Design review of the part built by this model. Coordinates are the model's own, in mm. Face numbers are marked on the shaded views. A direction names the side the tool comes from. Coordinates: 2 decimals unless noted, no trailing zeros. Write each loop counter-clockwise with the first axis right and the second up, starting at its lowest first coordinate (ties: lowest second). Pieces come first, ordered by that corner, then holes. Notation, with made-up numbers: (44.5, 50) -> (71.5, 50) arc R28 cw to (71.5, 71) -> close; hole circle Ø3 at (2.25, 44). An arc over 180 degrees is marked (long way). Write item = value, one per line. Start each with the question number.
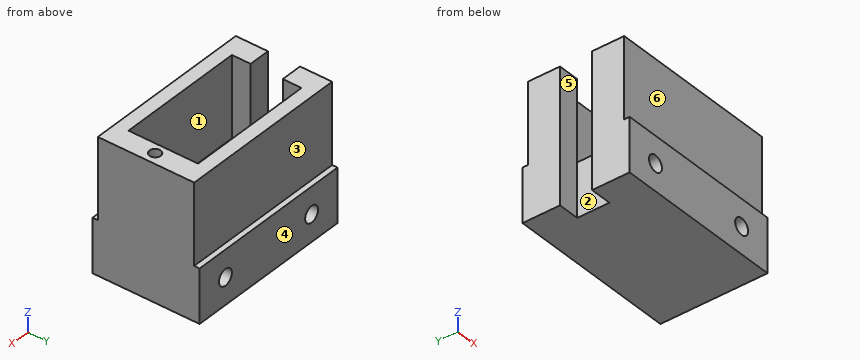
```python
from build123d import *

# Parameters (mm, degrees)
ESQUISSE15_W             = 32
ESQUISSE15_H             = 20
BOSS_EXTRU_1_DEPTH       = 10
ESQUISSE16_W             = 32
ESQUISSE16_H             = 18
ESQUISSE16_W_2           = 24
ESQUISSE16_H_2           = 13
BOSS_EXTRU_2_DEPTH       = 15
ESQUISSE17_W             = 25
ESQUISSE17_H             = 6
ENL_V_MAT_EXTRU_8_DEPTH  = 4
ESQUISSE19_R             = 1.05
ENL_V_MAT_EXTRU_10_DEPTH = 6
ENL_V_MAT_EXTRU_11_REACH = 22
ESQUISSE20_R             = 1.5


with BuildPart() as part:
    # Esquisse15 → Boss.-Extru.1 (new body)
    with BuildSketch(Plane.XY):
        Rectangle(ESQUISSE15_W, ESQUISSE15_H)
    extrude(amount=BOSS_EXTRU_1_DEPTH)

    # Esquisse16 → Boss.-Extru.2 (add)
    with BuildSketch(Plane.XY.offset(10)):
        Rectangle(ESQUISSE16_W, ESQUISSE16_H)
        Rectangle(ESQUISSE16_W_2, ESQUISSE16_H_2, mode=Mode.SUBTRACT)
    extrude(amount=BOSS_EXTRU_2_DEPTH)

    # Esquisse17 → Enlèv. mat.-Extru.8 (cut)
    with BuildSketch(Plane.ZY.offset(16)):
        with Locations((12.5, 0)):
            Rectangle(ESQUISSE17_W, ESQUISSE17_H)
    extrude(amount=-ENL_V_MAT_EXTRU_8_DEPTH, mode=Mode.SUBTRACT)

    # Esquisse19 → Enlèv. mat.-Extru.10 (cut)
    with BuildSketch(Plane.XY.offset(25)):
        with Locations((13.9, 0)):
            Circle(ESQUISSE19_R)
    extrude(amount=-ENL_V_MAT_EXTRU_10_DEPTH, mode=Mode.SUBTRACT)

    # Esquisse20 → Enlèv. mat.-Extru.11 (cut, up to next)
    with BuildSketch(Plane(origin=(0, 10, 0), x_dir=(1, 0, 0), z_dir=(0, 1, 0)), mode=Mode.PRIVATE) as enl_v_mat_extru_11_sk1:
        with Locations((-10, -5)):
            Circle(ESQUISSE20_R)
    enl_v_mat_extru_11_tool1 = extrude(enl_v_mat_extru_11_sk1.sketch, amount=-ENL_V_MAT_EXTRU_11_REACH, mode=Mode.PRIVATE) & part.part
    add(enl_v_mat_extru_11_tool1.solids().sort_by_distance((-10, 10, 5))[0], mode=Mode.SUBTRACT)
    # Esquisse20 → Enlèv. mat.-Extru.11 (cut, up to next)
    with BuildSketch(Plane(origin=(0, 10, 0), x_dir=(1, 0, 0), z_dir=(0, 1, 0)), mode=Mode.PRIVATE) as enl_v_mat_extru_11_sk2:
        with Locations((10, -5)):
            Circle(ESQUISSE20_R)
    enl_v_mat_extru_11_tool2 = extrude(enl_v_mat_extru_11_sk2.sketch, amount=-ENL_V_MAT_EXTRU_11_REACH, mode=Mode.PRIVATE) & part.part
    add(enl_v_mat_extru_11_tool2.solids().sort_by_distance((10, 10, 5))[0], mode=Mode.SUBTRACT)


solid = part.part
```
(1) For line 1 (X direction, y = -3.5, z = 5); line 2 (X direction, y = 1.5, z = 5); line 3 (Z direction, x = 10, y = 2.5), list the stretches that pass through material, from the lowest coordinate up.
(2) For the marked faces 1, 2 and 3, list the 3-axis set-ups (+Z, -Z, +X, -X, +Y, -Y) from which the entire face can be reached by the end or side of a thin tool; tool diameter is ignored.
(3) For pin 1 Ø10.5 at (x, y) = (-1, -0.5) entering from +Z; pin 2 Ø4.5 at (x, z) = (4, 19.5) entering from +Y; pin 3 Ø0.6 at (x, y) = (14, -0.5) entering from +Z, all flat-tipped, find the tip position at first contact; note any pin that passes through.
(4) Take a section at D-D, the plane z = 22.75. State the section outline as (x, y) points.
(5) Mouldability with a two-part tool opening along Y and no side actions: class the marked faces 4, 5 and 6 as pulls with the +Y half, pulls with the -Y half, needs draft (parallel to the pull), parting line crosses it, or undercut.
(6) Take a section at A-A, the plane z = 5. State the section outline as (x, y) points.
(7) Take a section at B-B, the plane x = -14. State the section outline as (y, z) points, then the cut area to 3 significant figures.
(8) Take a section at C-C, the plane y = 0. State the section outline as (x, z) points.
Report:
q1.line_1 = -16 to -11.5, -8.5 to 8.5, 11.5 to 16
q1.line_2 = -12 to -11.5, -8.5 to 8.5, 11.5 to 16
q1.line_3 = 0 to 3.5, 6.5 to 10
q2.face_1 = +Z
q2.face_2 = +Z, -Z, -X
q2.face_3 = +Z, +X, -X, +Y
q3.pin_1 = 10
q3.pin_2 = 9
q3.pin_3 = 19
q4.outline = (-16, -9) -> (16, -9) -> (16, 9) -> (-16, 9) -> (-16, 3) -> (-12, 3) -> (-12, 6.5) -> (12, 6.5) -> (12, -6.5) -> (-12, -6.5) -> (-12, -3) -> (-16, -3) -> close; hole circle Ø2.1 at (13.9, 0)
q5.face_4 = pulls with the +Y half
q5.face_5 = undercut
q5.face_6 = pulls with the -Y half
q6.outline = (-16, -10) -> (-11.5, -10) -> (-11.5, 10) -> (-16, 10) -> (-16, 3) -> (-12, 3) -> (-12, -3) -> (-16, -3) -> close; (-8.5, -10) -> (8.5, -10) -> (8.5, 10) -> (-8.5, 10) -> close; (11.5, -10) -> (16, -10) -> (16, 10) -> (11.5, 10) -> close
q7.outline = (-10, 0) -> (-3, 0) -> (-3, 25) -> (-9, 25) -> (-9, 10) -> (-10, 10) -> close; (3, 0) -> (10, 0) -> (10, 10) -> (9, 10) -> (9, 25) -> (3, 25) -> close
q7.area = 320 mm2
q8.outline = (-12, 0) -> (16, 0) -> (16, 25) -> (14.95, 25) -> (14.95, 19) -> (12.85, 19) -> (12.85, 25) -> (12, 25) -> (12, 10) -> (-12, 10) -> close; hole circle Ø3 at (-10, 5); hole circle Ø3 at (10, 5)
